Source: three-view drawing plus pictorial views. Frame: mm from the lowest corner of the part. A direction names the side the tool comes from. Round coordinates to 2 decimals unless told otherwise and drop trailing zeros. Loops run counter-clockwise (first coordinate to the right, second up) from the corner with the lowest first, then second, coordinate; pieces in that order, holes last. Notation, with made-up numbers: M 31.25,-12.75 L 68.25,-12.75 A17 cw 68.25,4.25 Z; hole C -6.5,40 d6. An arc over 180 degrees is marked long. Answer as a JSON object with one key per item and string values.
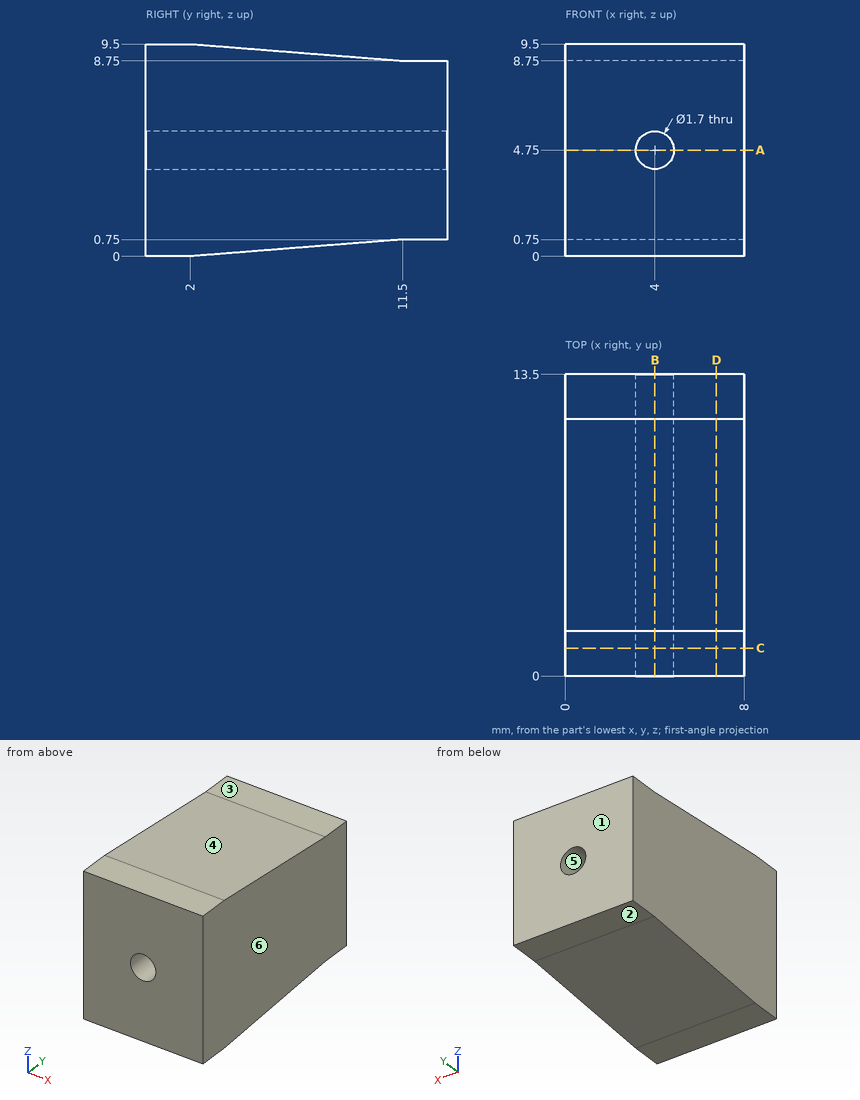
1) Cut plane B-B on x = 4. Return the cut outline in (y, z), and give its area (3 significant figures).
Geometry results:
{"outline": "M 0,0 L 2,0 L 11.5,0.75 L 13.5,0.75 L 13.5,3.9 L 0,3.9 Z; M 0,5.6 L 13.5,5.6 L 13.5,8.75 L 11.5,8.75 L 2,9.5 L 0,9.5 Z", "area": "95.2 mm2"}
2) Pull-direction query (X, two-part tool) for the marked faces 4, 5 and 6; classes: +X half, -X half, draft (parallel to the pull), parting line (faces both ways), or undercut.
Geometry results:
{"face 4": "draft", "face 5": "undercut", "face 6": "+X half"}
3) Line query: probe 1 along X at (y, z) = (8.75, 4.75); probe 2 along Z at (x, y) = (3.5, 3.5); probe 3 along X at (y, z) = (7.5, 4). Output: solid intervals per line, ascending.
Geometry results:
{"probe 1": "0 to 3.15, 4.85 to 8", "probe 2": "0.12 to 4.06, 5.44 to 9.38", "probe 3": "0 to 3.6, 4.4 to 8"}
4) Cut plane A-A on z = 4.75. Return the cut outline in (x, y).
Geometry results:
{"outline": "M 0,0 L 3.15,0 L 3.15,13.5 L 0,13.5 Z; M 4.85,0 L 8,0 L 8,13.5 L 4.85,13.5 Z"}
5) Set-up query: the marked faces 1, 2 and 3. Return all of +Z, -Z, +X, -X, +Y, -Y with unobstructed straight access to the full face (end or side cutting, diameter ignored); none if empty.
Geometry results:
{"face 1": "+Z, -Z, +X, -X, +Y", "face 2": "-Z, +X, -X, +Y", "face 3": "+Z, +X, -X, +Y"}
6) Cut plane D-D on x = 6.75. Return the cut outline in (y, z), and give its area (3 significant figures).
Geometry results:
{"outline": "M 0,0 L 2,0 L 11.5,0.75 L 13.5,0.75 L 13.5,8.75 L 11.5,8.75 L 2,9.5 L 0,9.5 Z", "area": "118 mm2"}
7) First-contact query: pin 1 (0.6 mm diameter, centred on x = 3.5, y = 12, fed in from +Z); pin 2 (2 mm diameter, centred on x = 2.5, z = 5, fed in from -Y); pin 3 (1.5 mm diameter, centred on x = 3.5, y = 7.5, fed in from +Z) (3 decimals); pin 4 (1 mm diameter, centred on x = 4, y = 12.5, fed in from -Z). Flat tips, straight axial feed; report the tip coordinate or a pass-through.
Geometry results:
{"pin 1": "z = 8.75", "pin 2": "y = 0", "pin 3": "z = 9.125", "pin 4": "z = 0.75"}
8) Cut plane C-C on y = 1.25. Return the cut outline in (x, z).
Geometry results:
{"outline": "M 0,0 L 8,0 L 8,9.5 L 0,9.5 Z; hole C 4,4.75 d1.7"}
